Can you work these out from the model? Positions are in its coordinate system, mm. A direction names the side the tool comes from. Coordinates: 2 decimals unless noted, no trailing zeros. Order: outer loops, then holes, each group sorted by start corner. A loop starts at its lowest first (then second) coordinate and runs counter-clockwise, first axis right, second up. Notation, with made-up numbers: (-38.5, 74.5) -> (5.5, 74.5) arc R11 ccw to (5.5, 86.5) -> close; hole circle Ø7 at (85.5, -4). An arc over 180 degrees is marked (long way). Answer as a JSON object with one key per item and string values. Group by question number.
(1) Which directions (+Z, -Z, +X, -X, +Y, -Y) give clear straight access to the entire face, cutting with the end or side of a thin tool? Please do faces 4 (the flat face through (-3, 592, -21.699)), 5 (the flat face through (-3, 592, -19.699)).
(2) For pin 1 (12 mm diameter, centred on x = -0.5, y = 690, fed in from -Z); pin 2 (10 mm diameter, centred on x = -4.5, y = 249.5, fed in from +Z), each with a flat end and sliding along its axis, tell me the tip position at first contact or that it passes through.
(3) I want a section at A-A, the plane z = -6.5. List the corners of the cut face in (x, y) for me.
(4) I need wall thicknesses on line 1 (Z direction, x = -11.25, y = 720); line 2 (X direction, y = 761.5, z = -23.5); line 3 (Z direction, x = -16, y = 1101). Which ranges of each line are inside material? Lowest first, please.
(5) I want a section at B-B, the plane x = -7. List the corners of the cut face in (y, z) for me, plus the area to 3 significant figures.
(6) If we mould it in two halves opening along X, with no side actions, what happens to faces 1 (the flat face through (-17.898, 592, -7)), 2 (the flat face through (11.102, 592, -7)), 3 (the flat face through (-4, 592, 8.301))? For each: pulls with the +X half, pulls with the -X half, needs draft (parallel to the pull), parting line crosses it, or undercut.
(7) I want a section at C-C, the plane y = 224. State how many separate pieces and enclosed holes the cut face has, plus the area to 3 significant figures.
Autodesk Inventor part; units mm, degrees
ref_plane "YZ Plane" through (0, 0, 0) normal (1, 0, 0) x (0, 1, 0)
ref_plane "XZ Plane" through (0, 0, 0) normal (0, 1, 0) x (-1, 0, 0)
ref_plane "XY Plane" through (0, 0, 0) normal (0, 0, 1) x (1, 0, 0)
sketch "Schizzo1" plane through (0, 0, 0) normal (0, 1, 0) x (-1, 0, 0)
  line L0 (14.898, -21.6987) -> (14.898, -31.6987)
  line L1 (-8.102, -21.6987) -> (-8.102, -31.6987)
  line L2 (-8.102, -31.6987) -> (-11.102, -31.6987)
  line L3 (-8.102, -21.6987) -> (14.898, -21.6987)
  line L4 (-10.3886, -19.6987) -> (17.0348, -19.6987)
  line L5 (14.898, -31.6987) -> (17.898, -31.6987)
  line L6 (17.898, -6.6987) -> (-17.7474, -6.6987) construction
  line L7 (-10.3886, 6.3013) -> (-10.3886, -19.6987)
  line L8 (17.0348, 6.3013) -> (-10.3886, 6.3013)
  line L9 (-10.3886, -19.6987) -> (17.0348, 6.3013) construction
  line L10 (17.0348, -19.6987) -> (-10.3886, 6.3013) construction
  line L11 (14.898, 8.3013) -> (-8.102, 8.3013)
  line L12 (-11.102, -31.6987) -> (-11.102, 18.3013)
  line L13 (17.898, -31.6987) -> (17.898, 18.3013)
  line L14 (-11.102, 18.3013) -> (-8.102, 18.3013)
  line L15 (14.898, 18.3013) -> (14.898, 8.3013)
  line L16 (17.898, 18.3013) -> (14.898, 18.3013)
  line L17 (17.0348, -19.6987) -> (17.0348, 6.3013)
  line L18 (-8.102, 18.3013) -> (-8.102, 8.3013)
  line L19 (17.2869, 17.8522) -> (15.509, 17.8522)
  line L20 (15.509, 17.8522) -> (15.509, 8.7505)
  line L21 (15.509, 8.7505) -> (17.2869, 8.7505)
  line L22 (17.2869, 8.7505) -> (17.2869, 17.8522)
  line L23 (17.2869, 17.8522) -> (15.509, 8.7505) construction
  line L24 (15.509, 17.8522) -> (17.2869, 8.7505) construction
  line L25 (17.2869, -22.1954) -> (15.509, -22.1954)
  line L26 (15.509, -22.1954) -> (15.509, -31.202)
  line L27 (15.509, -31.202) -> (17.2869, -31.202)
  line L28 (17.2869, -31.202) -> (17.2869, -22.1954)
  line L29 (17.2869, -22.1954) -> (15.509, -31.202) construction
  line L30 (15.509, -22.1954) -> (17.2869, -31.202) construction
  line L31 (-8.5206, -22.1954) -> (-10.6835, -22.1954)
  line L32 (-10.6835, -22.1954) -> (-10.6835, -31.202)
  line L33 (-10.6835, -31.202) -> (-8.5206, -31.202)
  line L34 (-8.5206, -31.202) -> (-8.5206, -22.1954)
  line L35 (-8.5206, -22.1954) -> (-10.6835, -31.202) construction
  line L36 (-10.6835, -22.1954) -> (-8.5206, -31.202) construction
  line L37 (-8.5206, 17.8522) -> (-10.6835, 17.8522)
  line L38 (-10.6835, 17.8522) -> (-10.6835, 8.7505)
  line L39 (-10.6835, 8.7505) -> (-8.5206, 8.7505)
  line L40 (-8.5206, 8.7505) -> (-8.5206, 17.8522)
  line L41 (-8.5206, 17.8522) -> (-10.6835, 8.7505) construction
  line L42 (-10.6835, 17.8522) -> (-8.5206, 8.7505) construction
  line L43 (-10.2389, 6.9058) -> (17.0348, 6.9058)
  line L44 (17.0348, 6.9058) -> (17.0348, 7.7637)
  line L45 (17.0348, 7.7637) -> (-10.2389, 7.7637)
  line L46 (-10.2389, 7.7637) -> (-10.2389, 6.9058)
  line L47 (-10.2389, 6.9058) -> (17.0348, 7.7637) construction
  line L48 (17.0348, 6.9058) -> (-10.2389, 7.7637) construction
  line L49 (-10.2389, -21.0418) -> (17.0348, -21.0418)
  line L50 (17.0348, -21.0418) -> (17.0348, -20.3019)
  line L51 (17.0348, -20.3019) -> (-10.2389, -20.3019)
  line L52 (-10.2389, -20.3019) -> (-10.2389, -21.0418)
  line L53 (-10.2389, -21.0418) -> (17.0348, -20.3019) construction
  line L54 (17.0348, -21.0418) -> (-10.2389, -20.3019) construction
  point P0 (0, 0)
  point P1 (0, 0)
  point P2 (3.3231, -6.6987)
  point P3 (16.398, 13.3013)
  point P4 (16.398, -26.6987)
  point P5 (-9.602, -26.6987)
  point P6 (-9.602, 13.3013)
  point P7 (3.398, 7.3347)
  point P8 (3.398, -20.6718)
  dimension "d0" = 50
  dimension "d1" = 23
  dimension "d2" = 3
  dimension "d3" = 10
  dimension "d4" = 10
  dimension "d5" = 10
  dimension "d6" = 2
  dimension "d7" = 2
extrude "Estrusione1" add sketch "Schizzo1" along normal blind 1200
properties part number "calcolo fem"
Computed values:
{
 "1": {"face 4": "-Z, +Y, -Y", "face 5": "+Y, -Y"},
 "2": {"pin 1": "stops at z = -21.7", "pin 2": "stops at z = 8.3"},
 "3": {"outline": "(-17.9, 0) -> (-17.03, 0) -> (-17.03, 1200) -> (-17.9, 1200) -> close; (10.39, 0) -> (11.1, 0) -> (11.1, 1200) -> (10.39, 1200) -> close"},
 "4": {"line 1": "z = -21.7 to -21.04, -20.3 to -19.7, 6.3 to 6.91, 7.76 to 8.3", "line 2": "x = -17.9 to -17.29, -15.51 to -14.9, 8.1 to 8.52, 10.68 to 11.1", "line 3": "z = -31.7 to -31.2, -22.2 to -21.04, -20.3 to -19.7, 6.3 to 6.91, 7.76 to 8.75, 17.85 to 18.3"},
 "5": {"outline": "(0, -21.7) -> (1200, -21.7) -> (1200, -21.04) -> (0, -21.04) -> close; (0, -20.3) -> (1200, -20.3) -> (1200, -19.7) -> (0, -19.7) -> close; (0, 6.3) -> (1200, 6.3) -> (1200, 6.91) -> (0, 6.91) -> close; (0, 7.76) -> (1200, 7.76) -> (1200, 8.3) -> (0, 8.3) -> close", "area": "2,880 mm2"},
 "6": {"face 1": "pulls with the -X half", "face 2": "pulls with the +X half", "face 3": "undercut"},
 "7": {"separate pieces": "1", "enclosed holes": "7", "area": "162 mm2"}
}
